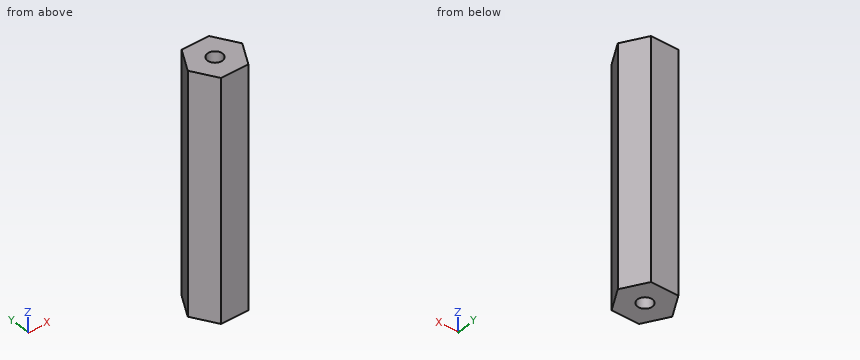
Autodesk Inventor part; units mm, degrees
ref_plane "YZ Plane" through (0, 0, 0) normal (1, 0, 0) x (0, 1, 0)
ref_plane "XZ Plane" through (0, 0, 0) normal (0, 1, 0) x (-1, 0, 0)
ref_plane "XY Plane" through (0, 0, 0) normal (0, 0, 1) x (1, 0, 0)
sketch "Sketch1" plane through (0, 0, 0) normal (0, 0, 1) x (1, 0, 0)
  line L0 (3.6662, -6.35) -> (-3.6662, -6.35)
  line L1 (-3.6662, -6.35) -> (-7.3323, 0)
  line L2 (-7.3323, 0) -> (-3.6662, 6.35)
  line L3 (-3.6662, 6.35) -> (3.6662, 6.35)
  line L4 (3.6662, 6.35) -> (7.3323, 0)
  line L5 (7.3323, 0) -> (3.6662, -6.35)
  point P0 (0, 0)
  point P1 (0, 0)
  dimension "d0" = 12.7
extrude "Extrusion1" add sketch "Sketch1" along normal blind 63.4492
sketch "Sketch2" plane through (0, 0, 63.4492) normal (0, 0, 1) x (1, 0, 0)
  point P0 (0, 0)
  point P1 (0, 0)
hole "Hole1" at (0, 0, 63.4492) direction (0, 0, -1) diameter 3.9624 depth 13.6144 tip angle 118
sketch "Sketch3" plane through (0, 0, 0) normal (0, 0, -1) x (-1, 0, 0)
  circle A0 centre (0, 0) radius 1.9812
hole "Hole2" at (0, 0, 0) direction (0, 0, 1) diameter 3.9624 depth 13.6144 tip angle 118
properties part number "STOCK,HEX,SHAFT,TURRET,ENCODER" material "Aluminum 6061"
Verification items for the finished model (mm, model axes). Give positions to 0.01 mm unless a question says otherwise; leave off trailing zeros. Order: outer loops, then holes, each group sorted by start corner. A loop starts at its lowest first (then second) coordinate and runs counter-clockwise, first axis right, second up. Notation, with made-up numbers: (33.25, 86.25) -> (57.25, 86.25) arc R27 ccw to (57.25, 123.25) -> close; hole circle Ø10 at (49.25, -10.75). An arc over 180 degrees is marked (long way). One line per item, written item: value.
(1) Sectioned sample at C-C on x = 6.5. Record the cut outline in (y, z), then the cut area to 3 significant figures.
Final values:
outline: (-1.44, 0) -> (1.44, 0) -> (1.44, 63.45) -> (-1.44, 63.45) -> close
area: 183 mm^2
(2) Sectioned sample at B-B on y = -5.5. Record the cut outline in (x, z), then the cut area to 3 significant figures.
Final values:
outline: (-4.16, 0) -> (4.16, 0) -> (4.16, 63.45) -> (-4.16, 63.45) -> close
area: 528 mm^2
(3) Scan lines: line 1 along X through (y, z) = (0, 58.5); line 2 along Y through (x, z) = (0, 9); line 3 along Y through (x, z) = (-1, 56.5). Record each from-to range of solid material in increasing order. Write a range as [from, to].
Final values:
line 1: [-7.33, -1.98], [1.98, 7.33]
line 2: [-6.35, -1.98], [1.98, 6.35]
line 3: [-6.35, -1.71], [1.71, 6.35]
(4) Sectioned sample at A-A on z = 44. Record the cut outline in (x, y).
Final values:
outline: (-7.33, 0) -> (-3.67, -6.35) -> (3.67, -6.35) -> (7.33, 0) -> (3.67, 6.35) -> (-3.67, 6.35) -> close
(5) Gauge pin test, flat ends, axial feed: pin 1 (1.5 mm diameter, centred on y = -2.5, z = 27, fed in from -X); pin 2 (3 mm diameter, centred on x = 0, y = 0, fed in from +Z); pin 3 (1.5 mm diameter, centred on x = 0.5, y = -1, fed in from -Z); pin 4 (3 mm diameter, centred on x = 3.5, y = -3.5, fed in from -Z). Record the tip position at first contact, or that the pin passes through.
Final values:
pin 1: x = -6.32
pin 2: z = 49.55
pin 3: z = 13.68
pin 4: z = 0
